The listing builds one solid part. Answer for the finished solid, in the listing's coordinates (mm). A direction names the side the tool comes from. Give positions to 0.01 mm unless a question says otherwise; leave off trailing zeros. Order: outer loops, then holes, each group sorted by start corner. A loop starts at its lowest first (then second) coordinate and runs counter-clockwise, first axis right, second up. Notation, with made-up numbers: (72, -18) - (89, -18) arc R26 cw to (89, 17) - close; hole circle Ø6 at (67.5, 31.25). An arc over 180 degrees is marked (long way). Use CSV: the item, a comma, the result in double quotes.
```python
from build123d import *

# Parameters (mm, degrees)
SKETCH2_R           = 1.35
BOSS_EXTRUDE2_DEPTH = 5
BOSS_EXTRUDE3_START = -5
SKETCH3_W           = 7
SKETCH3_H           = 8.5
SKETCH3_R           = 2.05
SKETCH3_W_2         = 8
BOSS_EXTRUDE3_DEPTH = 11
FILLET1_R           = 3
CHAMFER1_SIZE       = 6
CHAMFER2_SIZE2      = 6
CHAMFER2_SIZE       = 1
FILLET2_R           = 3
CHAMFER4_SIZE       = 6
CHAMFER5_SIZE2      = 6
CHAMFER5_SIZE       = 1
SKETCH4_W           = 8
SKETCH4_H           = 9
BOSS_EXTRUDE4_DEPTH = 8
SKETCH5_R           = 2.05
CUT_EXTRUDE1_DEPTH  = 9
SKETCH6_W           = 8
SKETCH6_H           = 8
BOSS_EXTRUDE5_DEPTH = 8
SKETCH7_R           = 2.05
CUT_EXTRUDE2_DEPTH  = 8
SKETCH8_W           = 8
SKETCH8_H           = 9
SKETCH8_H_2         = 8
CUT_EXTRUDE4_DEPTH  = 8
SKETCH9_W           = 8
SKETCH9_H           = 58
SKETCH9_H_2         = 43
SKETCH9_H_3         = 48
SKETCH9_W_2         = 52
SKETCH9_H_4         = 8
BOSS_EXTRUDE6_DEPTH = 5
SKETCH10_R          = 1.6
CUT_EXTRUDE5_DEPTH  = 153.761251631
FILLET3_R           = 2
CHAMFER6_SIZE       = 5


# Some blends are built 0.0001 mm under size
with BuildPart() as part:
    # Sketch2 → Boss-Extrude2 (new body)
    with BuildSketch(Plane.XY):
        Polygon((-35, -45), (67, -45), (76, -36), (76, 36), (67, 45), (-35, 45), (-35, 36), (68, 36), (68, -36), (-35, -36), align=None)
        with Locations((-31.5, -40.5)):
            Circle(SKETCH2_R, mode=Mode.SUBTRACT)
        with Locations((-31.5, 40.5)):
            Circle(SKETCH2_R, mode=Mode.SUBTRACT)
        with Locations((65.5, 40.5)):
            Circle(SKETCH2_R, mode=Mode.SUBTRACT)
        with Locations((65.5, -40.5)):
            Circle(SKETCH2_R, mode=Mode.SUBTRACT)
    extrude(amount=BOSS_EXTRUDE2_DEPTH)

    # Sketch3 → Boss-Extrude3 (add)
    # profile 1 of 2: a face of its own
    with BuildSketch(Plane.XY.offset(5).offset(BOSS_EXTRUDE3_START)):
        with Locations((-18, -31.75)):
            Rectangle(SKETCH3_W, SKETCH3_H)
        with Locations((-18, -31)):
            Circle(SKETCH3_R, mode=Mode.SUBTRACT)
    # profile 2 of 2: a face of its own
    with BuildSketch(Plane.XY.offset(5).offset(BOSS_EXTRUDE3_START)):
        with Locations((64, -31.75)):
            Rectangle(SKETCH3_W_2, SKETCH3_H)
        with Locations((64, -31)):
            Circle(SKETCH3_R, mode=Mode.SUBTRACT)
    boss_extrude3 = extrude(amount=BOSS_EXTRUDE3_DEPTH)

    # Fillet1
    fillet1_edges = [part.edges().sort_by_distance(p)[0] for p in [
        (-21.5, -27.5, 5.5),
        (-14.5, -27.5, 5.5),
        (68, -27.5, 8),
        (60, -27.5, 5.5),
    ]]
    fillet(fillet1_edges, radius=FILLET1_R)

    # Chamfer1
    chamfer1_edges = [part.edges().sort_by_distance(p)[0] for p in [
        (-18, -36, 5),
    ]]
    chamfer(chamfer1_edges, length=CHAMFER1_SIZE - 0.0001)  # a hair under: the kernel refuses the full size

    # Chamfer2
    chamfer2_edges = [part.edges().sort_by_distance(p)[0] for p in [
        (64, -36, 5),
    ]]
    chamfer2_side = [part.faces().sort_by_distance(p)[0] for p in [
        (64, -36.02, 5),
    ]]
    chamfer(chamfer2_edges, length=CHAMFER2_SIZE - 0.0001, length2=CHAMFER2_SIZE2 - 0.0001, reference=chamfer2_side[0])  # a hair under: the kernel refuses the full size

    # Mirror5: Boss-Extrude3 across plane
    add(boss_extrude3.mirror(Plane(origin=(0, 0, 0), x_dir=(0, 0, 1), z_dir=(0, -1, 0))))

    # Fillet2
    fillet2_edges = [part.edges().sort_by_distance(p)[0] for p in [
        (-21.5, 27.5, 5.5),
        (-14.5, 27.5, 5.5),
        (68, 27.5, 8),
        (60, 27.5, 5.5),
    ]]
    fillet(fillet2_edges, radius=FILLET2_R)

    # Chamfer4
    chamfer4_edges = [part.edges().sort_by_distance(p)[0] for p in [
        (-18, 36, 5),
    ]]
    chamfer(chamfer4_edges, length=CHAMFER4_SIZE - 0.0001)  # a hair under: the kernel refuses the full size

    # Chamfer5
    chamfer5_edges = [part.edges().sort_by_distance(p)[0] for p in [
        (64, 36, 5),
    ]]
    chamfer5_side = [part.faces().sort_by_distance(p)[0] for p in [
        (64, 36.02, 5),
    ]]
    chamfer(chamfer5_edges, length=CHAMFER5_SIZE - 0.0001, length2=CHAMFER5_SIZE2 - 0.0001, reference=chamfer5_side[0])  # a hair under: the kernel refuses the full size

    # Sketch4 → Boss-Extrude4 (add)
    with BuildSketch(Plane.XY.offset(5)):
        with Locations((-1, -40.5)):
            Rectangle(SKETCH4_W, SKETCH4_H)
        with Locations((32, -40.5)):
            Rectangle(SKETCH4_W, SKETCH4_H)
    boss_extrude4 = extrude(amount=BOSS_EXTRUDE4_DEPTH)

    # Sketch5 → Cut-Extrude1 (cut)
    with BuildSketch(Plane.XZ.offset(45)):
        with Locations(Location((-1, 9.5, 0), (0, 0, 270))):
            Circle(SKETCH5_R)
        with Locations(Location((32, 9.5, 0), (0, 0, 270))):
            Circle(SKETCH5_R)
    cut_extrude1 = extrude(amount=-CUT_EXTRUDE1_DEPTH, mode=Mode.SUBTRACT)

    # Mirror6: Boss-Extrude4, Cut-Extrude1 across plane
    add(boss_extrude4.mirror(Plane(origin=(0, 0, 0), x_dir=(0, 0, 1), z_dir=(0, -1, 0))))
    add(cut_extrude1.mirror(Plane(origin=(0, 0, 0), x_dir=(0, 0, 1), z_dir=(0, -1, 0))), mode=Mode.SUBTRACT)

    # Sketch6 → Boss-Extrude5 (add)
    with BuildSketch(Plane.XY.offset(5)):
        with Locations((72, 0)):
            Rectangle(SKETCH6_W, SKETCH6_H)
    extrude(amount=BOSS_EXTRUDE5_DEPTH)

    # Sketch7 → Cut-Extrude2 (cut)
    with BuildSketch(Plane(origin=(76, 0, 0), x_dir=(0, 0, -1), z_dir=(1, 0, 0))):
        with Locations(Location((-9.5, 0, 0), (0, 0, 90))):
            Circle(SKETCH7_R)
    extrude(amount=-CUT_EXTRUDE2_DEPTH, mode=Mode.SUBTRACT)

    # Sketch8 → Cut-Extrude4 (cut)
    with BuildSketch(Plane.XY.offset(5)):
        with Locations((-1, -40.5)):
            Rectangle(SKETCH8_W, SKETCH8_H)
        with Locations((32, -40.5)):
            Rectangle(SKETCH8_W, SKETCH8_H)
        with Locations((72, 0)):
            Rectangle(SKETCH8_W, SKETCH8_H_2)
        with Locations((32, 40.5)):
            Rectangle(SKETCH8_W, SKETCH8_H)
        with Locations((-1, 40.5)):
            Rectangle(SKETCH8_W, SKETCH8_H)
    extrude(amount=CUT_EXTRUDE4_DEPTH, mode=Mode.SUBTRACT)

    # Sketch9 → Boss-Extrude6 (add)
    with BuildSketch(Plane.XY.offset(5)):
        with Locations((0, -65)):
            Rectangle(SKETCH9_W, SKETCH9_H)
        with Locations((0, 65)):
            Rectangle(SKETCH9_W, SKETCH9_H)
        with Locations((45, 57.5)):
            Rectangle(SKETCH9_W, SKETCH9_H_2)
        with Locations((25, -60)):
            Rectangle(SKETCH9_W, SKETCH9_H_3)
        with Locations((94, 0)):
            Rectangle(SKETCH9_W_2, SKETCH9_H_4)
    extrude(amount=BOSS_EXTRUDE6_DEPTH)

    # Sketch10 → Cut-Extrude5 (cut, through all)
    with BuildSketch(Plane.XY.offset(10)):
        with Locations((0, -85)):
            Circle(SKETCH10_R)
        with Locations((0, 90)):
            Circle(SKETCH10_R)
        with Locations((45, 75)):
            Circle(SKETCH10_R)
        with Locations((116, 0)):
            Circle(SKETCH10_R)
        with Locations((25, -80)):
            Circle(SKETCH10_R)
    extrude(amount=-CUT_EXTRUDE5_DEPTH, mode=Mode.SUBTRACT)

    # Fillet3
    fillet3_edges = [part.edges().sort_by_distance(p)[0] for p in [
        (-4, -94, 7.5),
        (4, -94, 7.5),
        (-4, 94, 7.5),
        (4, 94, 7.5),
        (41, 79, 7.5),
        (49, 79, 7.5),
        (21, -84, 7.5),
        (29, -84, 7.5),
        (120, -4, 7.5),
        (120, 4, 7.5),
    ]]
    fillet(fillet3_edges, radius=FILLET3_R)

    # Chamfer6
    # the kernel refuses this chamfer: 5 mm, written as the material it adds along each edge
    with BuildSketch(Plane(origin=(21, -45, 5), x_dir=(-0.9996219169112968, 0, -0.027495876610586317), z_dir=(0, 1, 0)), Plane(origin=(-4, -45, 5), x_dir=(-0.9996219169112968, 0, -0.027495876610586327), z_dir=(0, 1, 0)), Plane(origin=(4, -36, 5), x_dir=(0.9996219169112968, 0, -0.027495876610586317), z_dir=(0, -1, 0)), Plane(origin=(29, -36, 5), x_dir=(0.9996219169112968, 0, -0.027495876610586337), z_dir=(0, -1, 0)), Plane(origin=(49, 36, 5), x_dir=(-0.027495876610586317, 0, 0.9996219169112968), z_dir=(0, 1, 0)), Plane(origin=(-4, 45, 5), x_dir=(0.027495876610586317, 0, 0.9996219169112968), z_dir=(0, -1, 0)), Plane(origin=(4, 36, 5), x_dir=(-0.027495876610586403, 0, 0.9996219169112968), z_dir=(0, 1, 0))) as chamfer6_piece_1:
        Polygon((CHAMFER6_SIZE * 0.999621916911, CHAMFER6_SIZE * 0.0274958766106), (-CHAMFER6_SIZE * 0.0274958766106, CHAMFER6_SIZE * 0.999621916911), (0, 0), align=None)
    extrude(amount=9)
    with BuildSketch(Plane(origin=(68, 4, 5), x_dir=(0, 0.9996219169112968, -0.027495876610586324), z_dir=(1, 0, 0)), Plane(origin=(76, -4, 5), x_dir=(0, -0.9996219169112968, -0.027495876610586324), z_dir=(-1, 0, 0))) as chamfer6_piece_2:
        Polygon((CHAMFER6_SIZE * 0.999621916911, CHAMFER6_SIZE * 0.0274958766106), (-CHAMFER6_SIZE * 0.0274958766106, CHAMFER6_SIZE * 0.999621916911), (0, 0), align=None)
    extrude(amount=8)
    with BuildSketch(Plane(origin=(41, 45, 5), x_dir=(-0.9996219169112968, 0, -0.027495876610586317), z_dir=(0, -1, 0))) as chamfer6_piece_3:
        Polygon((CHAMFER6_SIZE * 0.999621916911, -CHAMFER6_SIZE * 0.0274958766106), (-CHAMFER6_SIZE * 0.0274958766106, -CHAMFER6_SIZE * 0.999621916911), (0, 0), align=None)
    extrude(amount=9)


solid = part.part
```
Item 1: Find the intervals of material crossed by line 1 along Y through (x, z) = (0, 6.3); line 2 along X through (y, z) = (31, 7); line 3 along X through (y, z) = (31, 3.25), in increasing order.
Taken from the geometry:
line 1,"-94 to -86.6, -83.4 to -36, 36 to 88.4, 91.6 to 94"
line 2,"-21.5 to -20.05, -15.95 to -14.5, 60 to 61.95, 66.05 to 68"
line 3,"-21.5 to -20.05, -15.95 to -14.5, 60 to 61.95, 66.05 to 76"
Item 2: Each of these flat-tipped pins is pushed along its axis until it touches: pin 1 (11 mm diameter, centred on x = 50, y = -35, fed in from +Z); pin 2 (2.5 mm diameter, centred on y = -70, z = 8, fed in from +X); pin 3 (4 mm diameter, centred on y = 66, z = 8.5, fed in from -X); pin 4 (4 mm diameter, centred on y = -23.5, z = 7.5, fed in from -X). Where does it stop, or does it pass through?
Taken from the geometry:
pin 1,"z = 5"
pin 2,"x = 29"
pin 3,"x = -4"
pin 4,"through"
Item 3: The mould has two halves that part along Y. Classify faces 5 (the face through (-35, -40, 2)), 6 (the face through (62.5, 29.6, 5.4)), 7 (the face through (-18, -39, 8)), 8 (the face through (22, 36, 3)): +Y half, -Y half, draft (parallel to the pull), parting line (faces both ways), or undercut.
Taken from the geometry:
face 5,"draft"
face 6,"undercut"
face 7,"-Y half"
face 8,"undercut"
Item 4: The part is cut by section A-A (x = 31). Give the vertices of the cut face in (y, z), and give its area (3 significant figures).
Taken from the geometry:
outline,"(-45, 0) - (-36, 0) - (-36, 8) - (-45, 8) - close; (36, 0) - (45, 0) - (45, 5) - (36, 5) - close"
area,"117 mm^2"
Item 5: The part is cut by section D-D (z = 7.5). Count the separate pieces of the cut face and the enclosed holes in it, and give its area (3 significant figures).
Taken from the geometry:
separate pieces,"9"
enclosed holes,"9"
area,"2,490 mm^2"
Item 6: The part is cut by section C-C (x = 72). Give the vertices of the cut face in (y, z).
Taken from the geometry:
outline,"(-40, 0) - (40, 0) - (40, 5) - (9, 5) - (4, 10) - (-4, 10) - (-9, 5) - (-40, 5) - close"
Item 7: The part is cut by section B-B (y = -56.5). Give the vertices of the cut face in (x, z).
Taken from the geometry:
outline,"(-4, 5) - (4, 5) - (4, 10) - (-4, 10) - close; (21, 5) - (29, 5) - (29, 10) - (21, 10) - close"
Item 8: Which of the six approach directions +Z, -Z, +X, -X, +Y, -Y give full straight-line access (tool end or side, diameter ignored) to faces 1 (the face through (0, -69, 5)), 2 (the face through (18, -41, 7)), 3 (the face through (29, -64, 7)), 4 (the face through (-18, 39, 8))?
Taken from the geometry:
face 1,"-Z, +X, -X, -Y"
face 2,"+Z, +Y, -Y"
face 3,"+Z, -Z, +X, -Y"
face 4,"+Z, -X, +Y"
